Autodesk Inventor part; units mm, degrees
ref_plane "YZ Plane" through (0, 0, 0) normal (1, 0, 0) x (0, 1, 0)
ref_plane "XZ Plane" through (0, 0, 0) normal (0, 1, 0) x (-1, 0, 0)
ref_plane "XY Plane" through (0, 0, 0) normal (0, 0, 1) x (1, 0, 0)
sketch "Sketch1" plane through (0, 0, 0) normal (0, 0, 1) x (1, 0, 0)
  circle A0 centre (0, 0) radius 5.5
  circle A1 centre (6.2, 2.25) radius 0.5
  circle A2 centre (6.2, -2.25) radius 0.5
  line L0 (0, 0) -> (12.1327, 0) construction
  arc A3 (7.7, 2.25) -> (6.9352, 3.5575) centre (6.2, 2.25) ccw
  arc A4 (6.9352, -3.5575) -> (7.7, -2.25) centre (6.2, -2.25) ccw
  line L1 (3.1858, 5.6657) -> (6.9352, 3.5575)
  line L2 (3.1858, -5.6657) -> (6.9352, -3.5575)
  line L3 (7.7, -2.25) -> (7.7, 2.25)
  arc A5 (3.1858, 5.6657) -> (3.1858, -5.6657) centre (0, 0) ccw
  dimension "d1" = 11
  dimension "d12" = 1
  dimension "d13" = 1
  dimension "d14" = 4.5
  dimension "d16" = 3
  dimension "d17" = 3
  dimension "d18" = 6.2
  dimension "d19" = 6.5
extrude "Extrusion1" add sketch "Sketch1" along normal mid plane 2.5
sketch "Sketch2" plane through (0, 0, 0) normal (0, 0, 1) x (1, 0, 0)
  circle A0 centre (6.2, 2.25) radius 0.5
  circle A1 centre (6.2, -2.25) radius 0.5
  line L0 (8.15, 2.25) -> (8.15, -2.25) construction
  line L1 (5.1, 2.25) -> (5.1, -2.25)
  line L2 (11.2, -2.25) -> (11.2, 2.25)
  arc A2 (11.2, 2.25) -> (5.1, 2.25) centre (8.15, 2.25) ccw
  arc A3 (5.1, -2.25) -> (11.2, -2.25) centre (8.15, -2.25) ccw
  point P0 (0, 0)
  point P1 (8.15, 0)
  dimension "d20" = 1.1
  dimension "d21" = 5
extrude "Extrusion2" cut sketch "Sketch2" along normal mid plane 1
properties part number "double spring swivel 7"
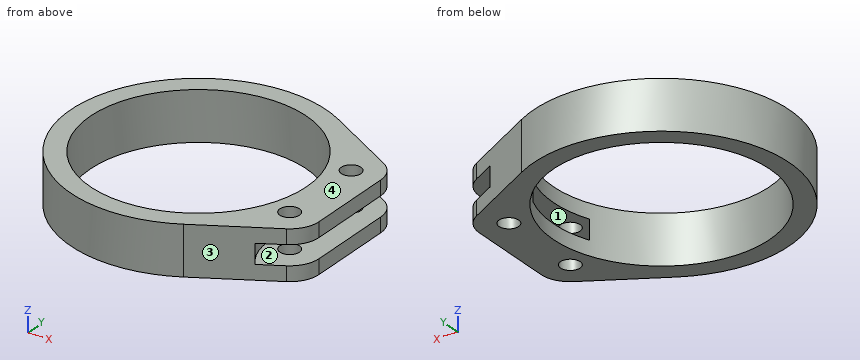
Part model, mm, in its own coordinate system. Face numbers are marked on the shaded views. Round coordinates to 2 decimals unless told otherwise and drop trailing zeros. Order: outer loops, then holes, each group sorted by start corner. A loop starts at its lowest first (then second) coordinate and runs counter-clockwise, first axis right, second up. Notation, with made-up numbers: (-26.75, 12) -> (-4.75, 12) arc R19 ccw to (-4.75, 42) -> close; hole circle Ø3 at (70.5, 83.25). An arc over 180 degrees is marked (long way). Put each result on its own line as item: value.
Q1. Pin check, flat tip, straight feed: pin 1 Ø1 at (x, z) = (-5, -0.5) entering from +Y. Stop position of the tip, or through.
From the geometry:
pin 1: stops at y = 4.69
Q2. Band-saw the part on D-D (z = -0.85). Give the cut face in (x, y), and give its area (3 significant figures).
From the geometry:
outline: (3.19, -5.67) -> (6.94, -3.56) arc R1.5 ccw to (7.7, -2.25) -> (7.7, 2.25) arc R1.5 ccw to (6.94, 3.56) -> (3.19, 5.67) arc R6.5 ccw (long way) to start; hole circle Ø11 at (0, 0); hole circle Ø1 at (6.2, -2.25); hole circle Ø1 at (6.2, 2.25)
area: 48.9 mm2
Q3. Band-saw the part on A-A (y = 0). Give the cut face in (x, z).
From the geometry:
outline: (-6.5, -1.25) -> (-5.5, -1.25) -> (-5.5, 1.25) -> (-6.5, 1.25) -> close; (5.5, -1.25) -> (7.7, -1.25) -> (7.7, -0.5) -> (5.5, -0.5) -> close; (5.5, 0.5) -> (7.7, 0.5) -> (7.7, 1.25) -> (5.5, 1.25) -> close
Q4. Pull direction Z, two halves, no side cores. Call the marked faces 1, 2, 3 and 4: pulls with the +Z half, pulls with the -Z half, needs draft (parallel to the pull), parting line crosses it, or undercut.
From the geometry:
face 1: undercut
face 2: undercut
face 3: needs draft
face 4: pulls with the +Z half
Q5. Band-saw the part on C-C (y = -3). Give the cut face in (x, z), and give its area (3 significant figures).
From the geometry:
outline: (-5.77, -1.25) -> (-4.61, -1.25) -> (-4.61, 1.25) -> (-5.77, 1.25) -> close; (4.61, -1.25) -> (7.5, -1.25) -> (7.5, -0.5) -> (5.19, -0.5) -> (5.19, 0.5) -> (7.5, 0.5) -> (7.5, 1.25) -> (4.61, 1.25) -> close
area: 7.81 mm2
Q6. Band-saw the part on B-B (x = 0). Give the cut face in (y, z), and give its area (3 significant figures).
From the geometry:
outline: (-6.5, -1.25) -> (-5.5, -1.25) -> (-5.5, 1.25) -> (-6.5, 1.25) -> close; (5.5, -1.25) -> (6.5, -1.25) -> (6.5, 1.25) -> (5.5, 1.25) -> close
area: 5.00 mm2
Q7. Wall check: line 1 (Z direction, x = 6, y = 3.5); line 2 (Y direction, x = 6, z = -0.6); line 3 (Y direction, x = 6.2, z = -1). Give the ranges that are in metal, low to high. Write a range as [from, to].
From the geometry:
line 1: z = [-1.25, -0.5], [0.5, 1.25]
line 2: y = [-4.08, -2.71], [-1.79, 1.79], [2.71, 4.08]
line 3: y = [-3.97, -2.75], [-1.75, 1.75], [2.75, 3.97]
